```python
from build123d import *

# Parameters (mm, degrees)
F1_DEPTH       = 6.35
F2_D           = 4.7625
F2_CSINK_D     = 12.7
F2_CSINK_ANGLE = 82


with BuildPart() as f1:
    # F0 (on Top) → F1 (new body)
    with BuildSketch(Plane.XY):
        with BuildLine():
            Line((-12.7, 15.875), (-12.7, -15.875))
            Line((-12.7, -15.875), (0, -15.875))
            Line((0, -15.875), (0, -13.49375))
            ThreePointArc((0, -13.49375), (-2.38125, -11.1125), (0, -8.73125))
            Line((0, -8.73125), (0, -3.175))
            ThreePointArc((0, -3.175), (-3.175, 0), (0, 3.175))
            Line((0, 3.175), (0, 8.73125))
            ThreePointArc((0, 8.73125), (-2.38125, 11.1125), (0, 13.49375))
            Line((0, 13.49375), (0, 15.875))
            Line((0, 15.875), (-12.7, 15.875))
        make_face()
        with BuildLine():
            Line((0, -13.49375), (0, -15.875))
            Line((0, -15.875), (12.7, -15.875))
            Line((12.7, -15.875), (12.7, 15.875))
            Line((12.7, 15.875), (0, 15.875))
            Line((0, 15.875), (0, 13.49375))
            ThreePointArc((0, 13.49375), (1.683798, 12.796298), (2.38125, 11.1125))
            ThreePointArc((2.38125, 11.1125), (1.683798, 9.428702), (0, 8.73125))
            Line((0, 8.73125), (0, 3.175))
            ThreePointArc((0, 3.175), (2.245064, 2.245064), (3.175, 0))
            ThreePointArc((3.175, 0), (2.245064, -2.245064), (0, -3.175))
            Line((0, -3.175), (0, -8.73125))
            ThreePointArc((0, -8.73125), (1.683798, -9.428702), (2.38125, -11.1125))
            ThreePointArc((2.38125, -11.1125), (1.683798, -12.796298), (0, -13.49375))
        make_face()
    extrude(amount=F1_DEPTH)

    # F2 (through all)
    with Locations(Plane(origin=(0, 0, 0), x_dir=(1, 0, 0), z_dir=(0, 0, -1))):
        with Locations((0, 11.1125), (0, -11.1125)):
            CounterSinkHole(F2_D / 2, F2_CSINK_D / 2, counter_sink_angle=F2_CSINK_ANGLE)


solid = f1.part
```
Geometry: final body of the model. Coordinates: model frame, mm. Coordinates: 2 decimals unless noted, no trailing zeros. Write each question's results on one line, items separated by ' | '.
(1) First-contact query: pin 1 Ø1.5 at (x, y) = (3.5, 0.5) entering from -Z. Flat tip, straight axial feed; report the tip coordinate or a pass-through.
Values found:
pin 1: stops at z = 0
(2) Section query A-A, the plane z = 5.5. Count the separate pieces of the cut face and the enclosed holes in it, plus the area to 3 significant figures.
Values found:
separate pieces: 1 | enclosed holes: 3 | area: 739 mm²
(3) Mould query, pull axis Y, two halves, no side actions, for faces 1 (the face through (0, 4, 0)), 2 (the face through (0.558, -8.6, 4.344)), 3 (the face through (0, -15.875, 3)). Classes: +Y half, -Y half, draft (parallel to the pull), parting line (faces both ways), or undercut.
Values found:
face 1: draft | face 2: undercut | face 3: -Y half
(4) Line query: line 1 (Y direction, x = 1, z = 4.25) (3 decimals); line 2 (Y direction, x = -1.25, z = 5.5) (3 decimals); line 3 (X direction, y = 14.5, z = 2). Output: solid intervals per line, ascending. Write a range as [from, to].
Values found:
line 1: y = [-15.875, -13.573], [-8.652, -3.013], [3.013, 8.652], [13.573, 15.875] | line 2: y = [-15.875, -13.139], [-9.086, -2.919], [2.919, 9.086], [13.139, 15.875] | line 3: x = [-12.7, -3.13], [3.13, 12.7]
